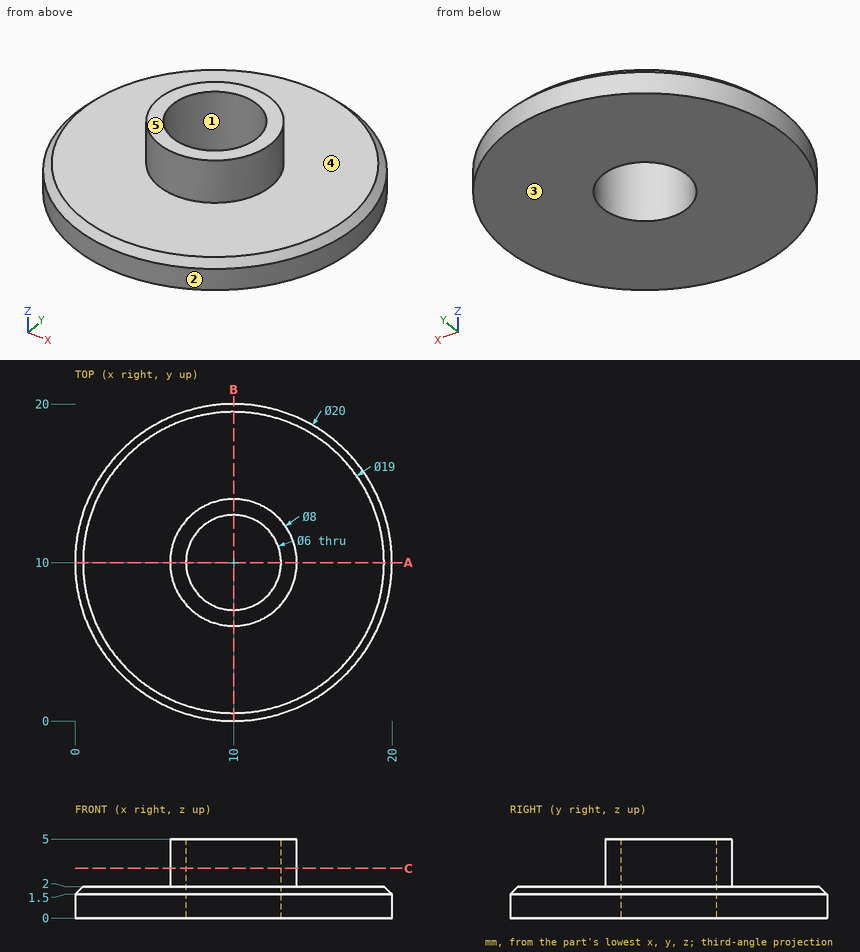
Design review of the part shown in the three views and the two pictorial views. Dimensions are in mm from the part's minimum x, y and z. A direction names the side the tool comes from. Round coordinates to 2 decimals unless told otherwise and drop trailing zeros. Order: outer loops, then holes, each group sorted by start corner. A loop starts at its lowest first (then second) coordinate and runs counter-clockwise, first axis right, second up.
(1) For P1, Ø1, axis at x = 7, y = 15, coming from the +Z side; P2, Ø3, axis at y = 7, z = 2, coming from the +X side, all flat-tipped, find the tip position at first contact; note any pin that passes through.
Working result:
P1: stops at z = 2
P2: stops at x = 19.87
(2) Take a section at A-A, the plane y = 10. State the section outline as (x, z) points.
Working result:
outline: (0, 0) - (7, 0) - (7, 5) - (6, 5) - (6, 2) - (0.5, 2) - (0, 1.5) - close; (13, 0) - (20, 0) - (20, 1.5) - (19.5, 2) - (14, 2) - (14, 5) - (13, 5) - close
(3) Take a section at C-C, the plane z = 3.15. State the section outline as (x, y) points, plus the area to 3 significant figures.
Working result:
outline: circle Ø8 at (10, 10); hole circle Ø6 at (10, 10)
area: 22.0 mm2
(4) Wall thickness on L1, parallel to Y at x = 10, z = 3.85; L2, parallel to Z at x = 6, y = 11.5; L3, parallel to Y at x = 7.5, z = 3: over which ranges is each line inside the solid? List them lowest first.
Working result:
L1: y = 6 to 7, 13 to 14
L2: z = 0 to 2
L3: y = 6.88 to 8.34, 11.66 to 13.12
(5) Tool access review of the marked faces 4 and 5: name each direction out of +Z, -Z, +X, -X, +Y, -Y from which nothing blocks a thin tool from reaching the whole face with its end or side.
Working result:
face 4: +Z
face 5: +Z, +X, -X, +Y, -Y
(6) Mouldability with a two-part tool opening along Y and no side actions: class the marked faces 1, 2 and 3 as released by +Y, released by -Y, zero draft, split by the parting line, or undercut.
Working result:
face 1: undercut
face 2: split by the parting line
face 3: zero draft
